Model file for the job. Use its own axes, mm. Face numbers are marked on the shaded views. Round coordinates to 2 decimals unless told otherwise and drop trailing zeros. Order: outer loops, then holes, each group sorted by start corner. A loop starts at its lowest first (then second) coordinate and runs counter-clockwise, first axis right, second up. Notation, with made-up numbers: M 81,20.5 L 109,20.5 A6 ccw 109,27.5 Z; hole C 80,44 d1. An arc over 180 degrees is marked long. Return JSON: item names as keys, results as strings. Group by question number.
Item 1: Pull direction X, two halves, no side cores. Call the marked faces 1 and 2: pulls with the +X half, pulls with the -X half, needs draft (parallel to the pull), parting line crosses it, or undercut.
Item 2: Probe line 1 along X through (y, z) = (3.25, 23); line 2 along Y through (x, z) = (-41.5, 50); line 3 along Z through (x, y) = (23.5, 9). List the from-to ranges inside material, lowest first.
Item 3: Slice it at B-B on z = 65.5. Write the cut outline in (x, y).
Item 4: Slice it at C-C on y = 4. Write the cut outline in (x, z).
Item 5: Pin check, flat tips, straight feed: pin 1 Ø3 at (x, z) = (-31, -29.5) entering from -Y; pin 2 Ø4 at (x, y) = (23.5, 10) entering from +Z. Stop position of each tip, or through.
Item 6: Slice it at A-A on x = -35. Write the cut outline in (y, z), then the cut area to 3 significant figures.
from build123d import *

# Parameters (mm, degrees)
BOSS_EXTRUDE1_DEPTH = 16
CUT_EXTRUDE1_START  = -1
CUT_EXTRUDE1_DEPTH  = 25
SKETCH5_R           = 2.000000000000003
CUT_EXTRUDE3_DEPTH  = 179.07652849266802
CUT_EXTRUDE4_DEPTH  = 179.07652849266802
FILLET1_R           = 1


with BuildPart() as part:
    # Sketch1 → Boss-Extrude1 (new body)
    with BuildSketch(Plane(origin=(0, 0, 0), x_dir=(1, 0, 0), z_dir=(0, 1, 0))):
        with BuildLine():
            Line((-48.499999999999986, 82.49999999999999), (48.500000000000014, 82.50000000000001))
            ThreePointArc((48.500000000000014, 82.50000000000001), (69.71320343559644, 73.71320343559644), (78.5, 52.500000000000014))
            Line((78.5, 52.500000000000014), (78.50000000000003, -82.5))
            Line((78.50000000000003, -82.5), (-78.49999999999997, -82.5))
            Line((-78.49999999999997, -82.5), (-78.5, 52.5))
            ThreePointArc((-78.5, 52.5), (-69.7132034355964, 73.71320343559643), (-48.499999999999986, 82.49999999999999))
        make_face()
    extrude(amount=BOSS_EXTRUDE1_DEPTH)

    # Sketch2 → Cut-Extrude1 (cut)
    with BuildSketch(Plane(origin=(0, 16, 0), x_dir=(1, 0, 0), z_dir=(0, 1, 0)).offset(CUT_EXTRUDE1_START)):
        with BuildLine():
            Line((-47.5, 81.5), (47.50000000000003, 81.50000000000003))
            ThreePointArc((47.50000000000003, 81.50000000000003), (68.71320343559645, 72.71320343559645), (77.50000000000003, 51.50000000000003))
            Line((77.50000000000003, 51.50000000000003), (77.50000000000004, -81.50000000000006))
            Line((77.50000000000004, -81.50000000000006), (77.50000000000006, -82.5))
            Line((77.50000000000006, -82.5), (75.39281372987732, -82.49999999999999))
            Line((75.39281372987732, -82.49999999999999), (-77.49999999999997, -82.5))
            Line((-77.49999999999997, -82.5), (-77.49999999999997, -81.49999999999997))
            Line((-77.49999999999997, -81.49999999999997), (-77.49999999999999, 51.500000000000014))
            ThreePointArc((-77.49999999999999, 51.500000000000014), (-68.71320343559641, 72.71320343559643), (-47.5, 81.5))
        make_face()
    extrude(amount=-CUT_EXTRUDE1_DEPTH, mode=Mode.SUBTRACT)

    # Sketch5 → Cut-Extrude3 (cut, through all)
    with BuildSketch(Plane.ZY.offset(78.49999999999999)):
        with Locations((-22.344222660164835, 4)):
            Circle(SKETCH5_R)
        with Locations((57.65577733983517, 4)):
            Circle(SKETCH5_R)
    extrude(amount=-CUT_EXTRUDE3_DEPTH, mode=Mode.SUBTRACT)

    # Sketch6 → Cut-Extrude4 (cut, through all)
    with BuildSketch(Plane.ZY.offset(78.49999999999999)):
        with BuildLine():
            ThreePointArc((82.49999999999999, 16), (78.51986342800406, 5.952610964746691), (69.49999999999999, -3.55e-15))
            Line((69.49999999999999, 0), (82.49999999999999, 0))
            Line((82.49999999999999, 0), (82.49999999999999, 16))
        make_face()
    extrude(amount=-CUT_EXTRUDE4_DEPTH, mode=Mode.SUBTRACT)

    # Fillet1
    # the kernel refuses this fillet: 1 mm, written as the material it takes off along each edge
    with BuildSketch(Plane(origin=(77.50000000000004, 0, 73.74999999999997), x_dir=(1, 0, -1.1e-16), z_dir=(-1.1e-16, 0, -1)), Plane(origin=(-77.49999999999997, 0, -51.5), x_dir=(-1, 0, 0), z_dir=(0, 0, 1))) as fillet1_piece_1:
        with BuildLine():
            CenterArc((FILLET1_R, -FILLET1_R), FILLET1_R, 90, 90)
            Line((0, -FILLET1_R), (0, 0))
            Line((0, 0), (FILLET1_R, 0))
        make_face()
    extrude(amount=125.25, mode=Mode.SUBTRACT)
    with BuildSketch(Plane(origin=(47.50000000000003, 0, -51.50000000000003), x_dir=(1, 0, 2.4e-16), z_dir=(-2.4e-16, 0, 1))) as fillet1_piece_2:
        with BuildLine():
            CenterArc((30 + FILLET1_R, FILLET1_R), FILLET1_R, 180, 90)
            Line((30, FILLET1_R), (30, 0))
            Line((30, 0), (30 + FILLET1_R, 0))
        make_face()
    revolve(axis=Axis((47.50000000000003, 0, -51.50000000000003), (0, 1, 0)), revolution_arc=90, mode=Mode.SUBTRACT)
    with BuildSketch(Plane(origin=(47.50000000000003, 0, -81.50000000000003), x_dir=(-3e-16, 0, -1), z_dir=(-1, 0, 3e-16))) as fillet1_piece_3:
        with BuildLine():
            CenterArc((FILLET1_R, -FILLET1_R), FILLET1_R, 90, 90)
            Line((0, -FILLET1_R), (0, 0))
            Line((0, 0), (FILLET1_R, 0))
        make_face()
    extrude(amount=95.00000000000003, mode=Mode.SUBTRACT)
    with BuildSketch(Plane(origin=(-47.499999999999986, 0, -51.5), x_dir=(-2.4e-16, 0, -1), z_dir=(1, 0, -2.4e-16))) as fillet1_piece_4:
        with BuildLine():
            CenterArc((30 + FILLET1_R, FILLET1_R), FILLET1_R, 180, 90)
            Line((30, FILLET1_R), (30, 0))
            Line((30, 0), (30 + FILLET1_R, 0))
        make_face()
    revolve(axis=Axis((-47.499999999999986, 0, -51.5), (0, 1, 0)), revolution_arc=89.99999999999994, mode=Mode.SUBTRACT)
    with BuildSketch(Plane(origin=(78.5, 0, -52.500000000000014), x_dir=(-1, 0, 2.1e-16), z_dir=(2.1e-16, 0, 1))) as fillet1_piece_5:
        with BuildLine():
            CenterArc((FILLET1_R, -FILLET1_R), FILLET1_R, 90, 90)
            Line((0, -FILLET1_R), (0, 0))
            Line((0, 0), (FILLET1_R, 0))
        make_face()
    extrude(amount=126.24999999999999, mode=Mode.SUBTRACT)
    with BuildSketch(Plane(origin=(48.50000000000004, 0, -52.50000000000006), x_dir=(-9.5e-16, 0, -1), z_dir=(-1, 0, 9.5e-16))) as fillet1_piece_6:
        with BuildLine():
            CenterArc((29.999999999999943 - FILLET1_R, -FILLET1_R), FILLET1_R, 1.272e-14, 90)
            Line((29.999999999999943, -FILLET1_R), (29.999999999999943, 0))
            Line((29.999999999999943, 0), (29.999999999999943 - FILLET1_R, 0))
        make_face()
    revolve(axis=Axis((48.50000000000004, 0, -52.50000000000006), (0, -1, 0)), revolution_arc=90.00000000000014, mode=Mode.SUBTRACT)
    with BuildSketch(Plane(origin=(-48.499999999999986, 0, -82.49999999999999), x_dir=(0, 1, 0), z_dir=(1, 0, -2.9e-16))) as fillet1_piece_7:
        with BuildLine():
            CenterArc((FILLET1_R, FILLET1_R), FILLET1_R, 180, 90)
            Line((-1.1e-16, FILLET1_R), (0, 0))
            Line((0, 0), (FILLET1_R, 0))
        make_face()
    extrude(amount=97, mode=Mode.SUBTRACT)
    with BuildSketch(Plane(origin=(-48.49999999999997, 0, -52.49999999999995), x_dir=(-1, 0, -1.66e-15), z_dir=(-1.66e-15, 0, 1))) as fillet1_piece_8:
        with BuildLine():
            CenterArc((30.00000000000003 - FILLET1_R, -FILLET1_R), FILLET1_R, 0, 90)
            Line((30.00000000000003 - FILLET1_R, 1.1e-16), (30.00000000000003, 0))
            Line((30.00000000000003, 0), (30.00000000000003, -FILLET1_R))
        make_face()
    revolve(axis=Axis((-48.49999999999997, 0, -52.49999999999995), (0, -1, 0)), revolution_arc=89.99999999999989, mode=Mode.SUBTRACT)
    with BuildSketch(Plane(origin=(-78.49999999999997, 16, 85), x_dir=(0, -1, 0), z_dir=(-2.1e-16, 0, -1))) as fillet1_piece_9:
        with BuildLine():
            CenterArc((FILLET1_R, -FILLET1_R), FILLET1_R, 90, 90)
            Line((0, -FILLET1_R), (0, 0))
            Line((0, 0), (FILLET1_R, 0))
        make_face()
    extrude(amount=137.5, mode=Mode.SUBTRACT)
    with BuildSketch(Plane(origin=(-48.49999999999997, 16, -52.49999999999995), x_dir=(-1, 0, -1.66e-15), z_dir=(-1.66e-15, 0, 1))) as fillet1_piece_10:
        with BuildLine():
            CenterArc((30.00000000000003 - FILLET1_R, FILLET1_R), FILLET1_R, 270, 90)
            Line((30.00000000000003 - FILLET1_R, 0), (30.00000000000003, 0))
            Line((30.00000000000003, 0), (30.00000000000003, FILLET1_R))
        make_face()
    revolve(axis=Axis((-48.49999999999997, 16, -52.49999999999995), (0, -1, 0)), revolution_arc=89.99999999999989, mode=Mode.SUBTRACT)
    with BuildSketch(Plane(origin=(-48.499999999999986, 16, -82.49999999999999), x_dir=(0, -1, 0), z_dir=(1, 0, -2.9e-16))) as fillet1_piece_11:
        with BuildLine():
            CenterArc((FILLET1_R, -FILLET1_R), FILLET1_R, 90, 90)
            Line((0, -FILLET1_R), (0, 0))
            Line((0, 0), (FILLET1_R, 0))
        make_face()
    extrude(amount=97, mode=Mode.SUBTRACT)
    with BuildSketch(Plane(origin=(48.50000000000004, 16, -52.50000000000006), x_dir=(-9.5e-16, 0, -1), z_dir=(-1, 0, 9.5e-16))) as fillet1_piece_12:
        with BuildLine():
            CenterArc((29.999999999999943 - FILLET1_R, FILLET1_R), FILLET1_R, 270, 90)
            Line((29.999999999999943, FILLET1_R), (29.999999999999943, 0))
            Line((29.999999999999943, 0), (29.999999999999943 - FILLET1_R, 0))
        make_face()
    revolve(axis=Axis((48.50000000000004, 16, -52.50000000000006), (0, -1, 0)), revolution_arc=90.00000000000014, mode=Mode.SUBTRACT)
    with BuildSketch(Plane(origin=(78.5, 16, -52.500000000000014), x_dir=(-1, 0, 2.1e-16), z_dir=(2.1e-16, 0, 1))) as fillet1_piece_13:
        with BuildLine():
            CenterArc((FILLET1_R, FILLET1_R), FILLET1_R, 180, 90)
            Line((0, FILLET1_R), (0, 0))
            Line((0, 0), (FILLET1_R, 0))
        make_face()
    extrude(amount=137.5, mode=Mode.SUBTRACT)
    with BuildSketch(Plane(origin=(-78.49999999999997, 0, 73.75), x_dir=(0, 1, 0), z_dir=(-2.1e-16, 0, -1))) as fillet1_piece_14:
        with BuildLine():
            CenterArc((FILLET1_R, FILLET1_R), FILLET1_R, 180, 90)
            Line((-1.1e-16, FILLET1_R), (0, 0))
            Line((0, 0), (FILLET1_R, 0))
        make_face()
    extrude(amount=126.25, mode=Mode.SUBTRACT)
    with BuildSketch(Plane(origin=(81.35302601856634, 16, 82.5), x_dir=(0, 0, -1), z_dir=(-1, 0, 0))) as fillet1_piece_15:
        with BuildLine():
            CenterArc((1.1090314143661004, 1), FILLET1_R, 172.23715283019968, 97.76284716980035)
            ThreePointArc((0.11819577889333743, 1.135073104196561), (0.05009298550456265, 0.5684742376371492), (0, 0))
            Line((0, 0), (1.1090314143661004, 0))
        make_face()
    extrude(amount=162.70605203713265, mode=Mode.SUBTRACT)


solid = part.part
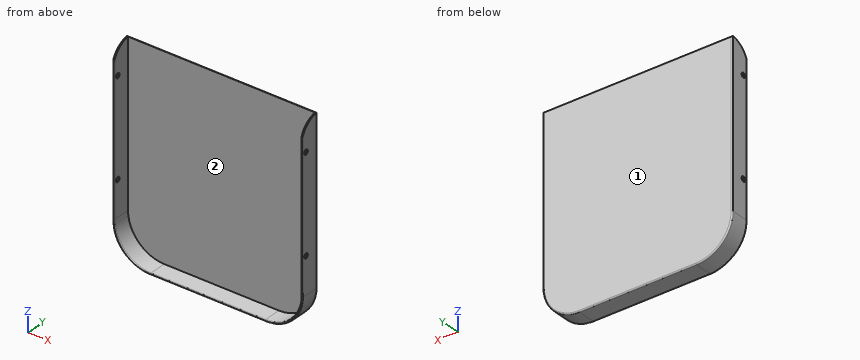
Output values:
{
 "1": {"face 1": "needs draft", "face 2": "undercut"},
 "2": {"line 1": "-78.5 to -77.5, 77.5 to 78.5", "line 2": "15 to 16", "line 3": "-82.5 to -81.5"},
 "3": {"outline": "M -78.5,1 A1 ccw -78,0.13 A1 ccw -77.5,1 L -77.5,15 L 77.5,15 L 77.5,1 A1 ccw 78,0.13 A1 ccw 78.5,1 L 78.5,15 A1 ccw 77.5,16 L -77.5,16 A1 ccw -78.5,15 Z"},
 "4": {"outline": "M -78.5,-52.5 A30 ccw -48.5,-82.5 L 48.5,-82.5 A30 ccw 78.5,-52.5 L 78.5,-24.34 L 77.5,-24.34 L 77.5,-51.5 A30 cw 47.5,-81.5 L -47.5,-81.5 A30 cw -77.5,-51.5 L -77.5,-24.34 L -78.5,-24.34 Z; M -78.5,-20.34 L -77.5,-20.34 L -77.5,55.66 L -78.5,55.66 Z; M -78.5,59.66 L -77.5,59.66 L -77.5,76.67 L -78.5,76.67 Z; M 77.5,-20.34 L 78.5,-20.34 L 78.5,55.66 L 77.5,55.66 Z; M 77.5,59.66 L 78.5,59.66 L 78.5,76.67 L 77.5,76.67 Z"},
 "5": {"pin 1": "y = 15", "pin 2": "z = -81.5"},
 "6": {"outline": "M 0.13,-82 A1 ccw 1,-82.5 L 15,-82.5 A1 ccw 16,-81.5 L 16,81.39 A1 ccw 15,82.39 L 15,-81.5 L 1,-81.5 A1 ccw Z", "area": "179 mm²"}
}
